Design review of the part shown in the three views and the two pictorial views. Dimensions are in mm from the part's minimum x, y and z. A direction names the side the tool comes from. Round coordinates to 2 decimals unless told otherwise and drop trailing zeros. Loops run counter-clockwise (first coordinate to the right, second up) from the corner with the lowest first, then second, coordinate; pieces in that order, holes last. Notation, with made-up numbers: M 46,64 L 80,64 A32 ccw 80,92 Z; hole C 81,78.5 d6. An arc over 180 degrees is marked long. One line per question, with ' | ' between items. Start each with the question number.
1) For probe 1 along X at (y, z) = (546.5, 420.5); probe 2 along Y at (x, z) = (250, 217); probe 3 along X at (y, z) = (72.5, 181) (1 decimal), list the stretches that pass through material, from the lowest coordinate up. Write a range as from..to.
2) We need section C-C (y = 311). Give the boundary of the cut face in (x, z), and give its area (3 significant figures).
3) Mouldability with a two-part tool opening along X and no side actions: class the marked faces 4, 5 and 6 as pulls with the +X half, pulls with the -X half, needs draft (parallel to the pull), parting line crosses it, or undercut.
4) We need section A-A (y = 162). Give the boundary of the cut face in (x, z) (1 decimal).
5) We need section D-D (x = 508). Give the boundary of the cut face in (y, z), and give its area (3 significant figures).
6) For pin 1 Ø12 at (x, z) = (518, 115) entering from -Y, flat-tipped, find the tip position at first contact; note if it passes through.
7) We need section B-B (z = 455.5). Give the boundary of the cut face in (x, y) (1 decimal), and give its area (3 significant figures).
8) For the marked faces 1, 2 and 3, list the 3-axis set-ups (+Z, -Z, +X, -X, +Y, -Y) from which the entire face can be reached by the end or side of a thin tool; tool diameter is ignored.
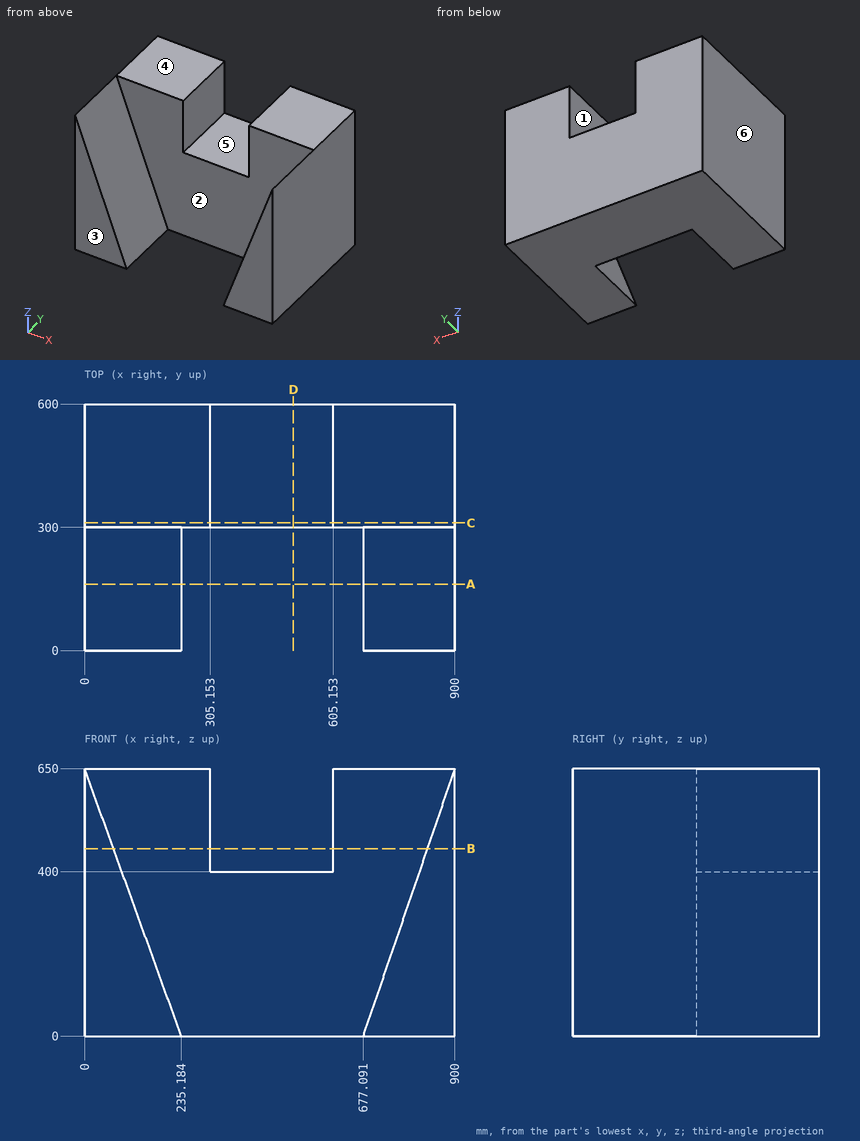
Answers below:
1) probe 1: 0..305.15, 605.15..900 | probe 2: 300..600 | probe 3: 0..169.7, 739.2..900
2) outline: M 0,0 L 900,0 L 900,650 L 605.15,650 L 605.15,400 L 305.15,400 L 305.15,650 L 0,650 Z | area: 510,000 mm^2
3) face 4: needs draft | face 5: undercut | face 6: pulls with the -X half
4) outline: M 0,0 L 235.2,0 L 0,650 Z; M 677.1,0 L 900,0 L 900,650 Z
5) outline: M 300,0 L 600,0 L 600,400 L 300,400 Z | area: 120,000 mm^2
6) pin 1: y = 300
7) outline: M 0,0 L 70.4,0 L 70.4,300 L 305.2,300 L 305.2,600 L 0,600 Z; M 605.2,300 L 833.3,300 L 833.3,0 L 900,0 L 900,600 L 605.2,600 Z | area: 221,000 mm^2
8) face 1: +Z, +Y, -Y | face 2: +Z, -Y | face 3: +Z, -Z, +X, -X, -Y
